from build123d import *

# Parameters (mm, degrees)
SKETCH1_W               = 30
SKETCH1_H               = 25
BOSS_EXTRUDE1_DEPTH     = 10
SKETCH2_W               = 50
SKETCH2_H               = 5
BOSS_EXTRUDE2_DEPTH     = 10
CUT_EXTRUDE1_DEPTH      = 49.218253805
CUT_EXTRUDE1_DEPTH_BACK = 49.218253805
SKETCH3_W               = 20
SKETCH3_H               = 15


with BuildPart() as part:
    # Sketch1 → Boss-Extrude1 (new body)
    with BuildSketch(Plane.XY):
        with Locations((15, 12.5)):
            Rectangle(SKETCH1_W, SKETCH1_H)
    extrude(amount=BOSS_EXTRUDE1_DEPTH)

    # Sketch2 → Boss-Extrude2 (add)
    with BuildSketch(Plane.XY.offset(10)):
        with Locations((15, 2.5)):
            Rectangle(SKETCH2_W, SKETCH2_H)
    extrude(amount=-BOSS_EXTRUDE2_DEPTH)

    # Sketch3 → Cut-Extrude1 (cut, two sides: drawn at the far end of the back side and taken through both)
    with BuildSketch(Plane.XY.offset(10).offset(-CUT_EXTRUDE1_DEPTH_BACK)):
        with Locations((15, 12.5)):
            Rectangle(SKETCH3_W, SKETCH3_H)
    extrude(amount=CUT_EXTRUDE1_DEPTH + CUT_EXTRUDE1_DEPTH_BACK, mode=Mode.SUBTRACT)


solid = part.part
For this review, take the finished solid that the model builds, in its own axes (mm). A direction names the side the tool comes from. Round coordinates to 2 decimals unless told otherwise and drop trailing zeros. Loops run counter-clockwise (first coordinate to the right, second up) from the corner with the lowest first, then second, coordinate; pieces in that order, holes last. Notation, with made-up numbers: (19, -37) - (49, -37) arc R7 cw to (49, -26) - close; hole circle Ø3 at (65.25, 30). An arc over 180 degrees is marked (long way). One line per item, written item: value. Start each with the question number.
Item 1: The part is to be moulded in two halves that separate along Y. For faces 5 (the flat face through (-10, 2, 5)), 6 (the flat face through (15, 25, 5)), 7 (the flat face through (25, 12, 5)), 8 (the flat face through (15, 0, 5)), say which applies: +Y half, -Y half, draft (parallel to the pull), parting line (faces both ways), or undercut.
Item 2: Take a section at C-C (z = 5.75). Give the boundary of the cut face in (x, y).
Item 3: Take a section at A-A (x = 23.5). Give the boundary of the cut face in (y, z), plus the area to 3 significant figures.
Item 4: Take a section at B-B (y = 7.5). Give the boundary of the cut face in (x, z), plus the area to 3 significant figures.
Item 5: For L1, parallel to Y at x = 13, z = 4.5; L2, parallel to X at y = 18.25, z = 3; L3, parallel to X at y = 24.25, z = 4.5, list the stretches that pass through material, from the lowest coordinate up.
Item 6: Take a section at D-D (x = 34). Give the boundary of the cut face in (y, z).
Item 7: Clearance check with flat-ended pins moving along their axes: pin 1 Ø4 at (y, z) = (16, 1.5) entering from +X; pin 2 Ø5 at (x, z) = (36, 5.5) entering from +Y. State where each tip first meets the part, or that it passes through.
Item 8: For faces 1 (the flat face through (35, 5, 5)), 2 (the flat face through (15, 4, 0)), 3 (the flat face through (15, 20, 5)), 4 (the flat face through (0, 15, 5)), list the 3-axis set-ups (+Z, -Z, +X, -X, +Y, -Y) from which the entire face can be reached by the end or side of a thin tool; tool diameter is ignored.
Answer below:
1. face 5: draft
1. face 6: +Y half
1. face 7: undercut
1. face 8: -Y half
2. outline: (-10, 0) - (40, 0) - (40, 5) - (30, 5) - (30, 25) - (0, 25) - (0, 5) - (-10, 5) - close; hole (5, 5) - (25, 5) - (25, 20) - (5, 20) - close
3. outline: (0, 0) - (5, 0) - (5, 10) - (0, 10) - close; (20, 0) - (25, 0) - (25, 10) - (20, 10) - close
3. area: 100 mm2
4. outline: (0, 0) - (5, 0) - (5, 10) - (0, 10) - close; (25, 0) - (30, 0) - (30, 10) - (25, 10) - close
4. area: 100 mm2
5. L1: y = 0 to 5, 20 to 25
5. L2: x = 0 to 5, 25 to 30
5. L3: x = 0 to 30
6. outline: (0, 0) - (5, 0) - (5, 10) - (0, 10) - close
7. pin 1: stops at x = 30
7. pin 2: stops at y = 5
8. face 1: +Z, -Z, +X, +Y
8. face 2: -Z, +X, -X, +Y, -Y
8. face 3: +Z, -Z
8. face 4: +Z, -Z, -X, +Y
